Work out the finished part from the listing and answer in its coordinate system (mm). Face numbers are marked on the shaded views. A direction names the side the tool comes from. Coordinates: 2 decimals unless noted, no trailing zeros. Loops run counter-clockwise (first coordinate to the right, second up) from the corner with the lowest first, then second, coordinate; pieces in that order, holes last. Notation, with made-up numbers: (23, 51) -> (66, 51) arc R24 cw to (66, 85) -> close; hole circle Ø3 at (-30.75, -1.5). An arc over 180 degrees is marked (long way). One line per question, with ' | ' between items.
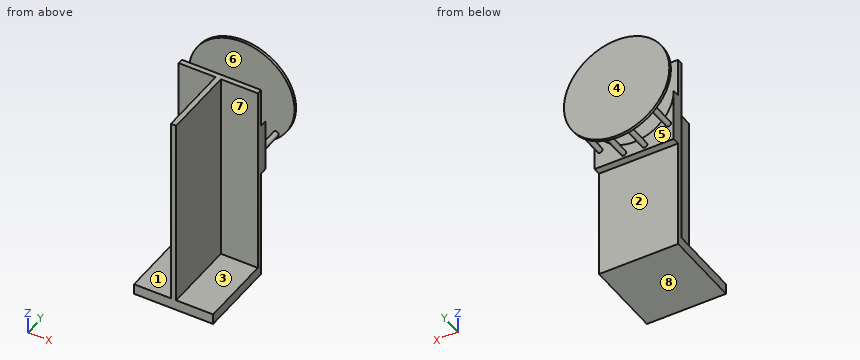
```python
from build123d import *

# Parameters (mm, degrees)
F0_W      = 38.1
F0_H      = 38.1
F1_DEPTH  = 5.08
F3_DEPTH  = 92.71
F5_DEPTH  = 3.4798
F7_R      = 25.4
F8_DEPTH  = 1.27
F9_R      = 1.27
F10_DEPTH = 12.7


with BuildPart() as f1:
    # F0 (on Top) → F1 (new body)
    with BuildSketch(Plane.XY):
        Rectangle(F0_W, F0_H)
    extrude(amount=F1_DEPTH)

    # F2 (on face) → F3 (join)
    with BuildSketch(Plane.XY.offset(5.08)):
        Polygon((19.05, 19.05), (1.27, 19.05), (-1.27, 19.05), (-19.05, 19.05), (-19.05, 16.51), (-1.27, 16.51), (-1.27, -19.05), (1.27, -19.05), (1.27, 16.51), (19.05, 16.51), align=None)
    extrude(amount=F3_DEPTH)

    # F4 (on face) → F5 (join)
    with BuildSketch(Plane(origin=(0, 19.05, 0), x_dir=(-1, 0, 0), z_dir=(0, 1, 0))):
        with BuildLine():
            ThreePointArc((19.05, 78.74), (0, 59.69), (-19.05, 78.74))
            Line((-19.05, 78.74), (-19.05, 59.69))
            Line((-19.05, 59.69), (-19.05, 53.34))
            Line((-19.05, 53.34), (19.05, 53.34))
            Line((19.05, 53.34), (19.05, 59.69))
            Line((19.05, 59.69), (19.05, 78.74))
        make_face()
    extrude(amount=F5_DEPTH)



with BuildPart() as f8:
    # F7 (on offset) → F8 (new body)
    with BuildSketch(Plane(origin=(0, 35.2298, 0), x_dir=(-1, 0, 0), z_dir=(0, 1, 0))):
        with Locations((0, 78.74)):
            Circle(F7_R)
    extrude(amount=F8_DEPTH)


with BuildPart() as f1_1:
    add(f1.part)

    add(f8.part)  # F10 merges F8
    # F9 (on face) → F10 (join, through all)
    with BuildSketch(Plane(origin=(0, 22.5298, 0), x_dir=(-1, 0, 0), z_dir=(0, 1, 0))):
        with Locations((-5.08, 55.88)):
            Circle(F9_R)
        with Locations((5.08, 55.88)):
            Circle(F9_R)
        with Locations((-16.51, 62.23)):
            Circle(F9_R)
        with Locations((16.51, 62.23)):
            Circle(F9_R)
    extrude(amount=F10_DEPTH)


solid = f1_1.part
```
1) Flat-ended cylindrical pins translate along their axes: pin 1 (21 mm diameter, centred on y = 10.5, z = 25, fed in from -X); pin 2 (11.5 mm diameter, centred on x = -2.5, y = 6.5, fed in from +Z); pin 3 (2 mm diameter, centred on y = 0, z = 33, fed in from +X). Find the tip coordinate at first contact, or state that the pin passes through.
Check values:
pin 1: stops at x = -19.05 | pin 2: stops at z = 97.79 | pin 3: stops at x = 1.27
2) Find the intervals of material crossed by line 1 along Y through (x, z) = (-10.5, 86); line 2 along Y through (x, z) = (-0.5, 97); line 3 along Z through (x, y) = (-1.5, 15), in increasing order.
Check values:
line 1: y = 16.51 to 19.05, 35.23 to 36.5 | line 2: y = -19.05 to 19.05, 35.23 to 36.5 | line 3: z = 0 to 5.08
3) Find section A-A (z = 76.5). Write down the section's boundary in (x, y), plus the area to 3 significant figures.
Check values:
outline: (-25.3, 35.23) -> (25.3, 35.23) -> (25.3, 36.5) -> (-25.3, 36.5) -> close; (-19.05, 16.51) -> (-1.27, 16.51) -> (-1.27, -19.05) -> (1.27, -19.05) -> (1.27, 16.51) -> (19.05, 16.51) -> (19.05, 22.53) -> (18.92, 22.53) -> (18.92, 19.05) -> (-18.92, 19.05) -> (-18.92, 22.53) -> (-19.05, 22.53) -> close | area: 252 mm^2
4) Find section D-D (z = 25). Write down the section's boundary in (x, y), plus the area to 3 significant figures.
Check values:
outline: (-19.05, 16.51) -> (-1.27, 16.51) -> (-1.27, -19.05) -> (1.27, -19.05) -> (1.27, 16.51) -> (19.05, 16.51) -> (19.05, 19.05) -> (-19.05, 19.05) -> close | area: 187 mm^2
5) For the marked faces 1, 2, 3 and 4, determine the directions among +Z, -Z, +X, -X, +Y, -Y from which every point of the face is accessible in a straight line to the end or side of a thin tool.
Check values:
face 1: +Z, -X, -Y | face 2: -Z, +X, -X, +Y | face 3: +Z, +X, -Y | face 4: +Z, -Z, +X, -X, +Y
6) Find section C-C (y = -13). Write down the section's boundary in (x, z), plus the area to 3 significant figures.
Check values:
outline: (-19.05, 0) -> (19.05, 0) -> (19.05, 5.08) -> (1.27, 5.08) -> (1.27, 97.79) -> (-1.27, 97.79) -> (-1.27, 5.08) -> (-19.05, 5.08) -> close | area: 429 mm^2
7) Find section B-B (x = 9.5). Write down the section's boundary in (y, z), plus the area to 3 significant figures.
Check values:
outline: (-19.05, 0) -> (19.05, 0) -> (19.05, 53.34) -> (22.53, 53.34) -> (22.53, 62.23) -> (19.05, 62.23) -> (19.05, 97.79) -> (16.51, 97.79) -> (16.51, 5.08) -> (-19.05, 5.08) -> close; (35.23, 55.18) -> (36.5, 55.18) -> (36.5, 102.3) -> (35.23, 102.3) -> close | area: 520 mm^2
8) The mould has two halves that part along Y. Classify the marked faces 5, 6, 7 and 8: released by +Y, released by -Y, zero draft, split by the parting line, or undercut.
Check values:
face 5: undercut | face 6: undercut | face 7: released by -Y | face 8: zero draft
